Geometry: final body of the model. Coordinates: model frame, mm. Round coordinates to 2 decimals unless told otherwise and drop trailing zeros. Loops run counter-clockwise (first coordinate to the right, second up) from the corner with the lowest first, then second, coordinate; pieces in that order, holes last. Notation, with made-up numbers: M -33.75,-16 L 0.25,-16 A8 cw 0.25,-5 Z; hole C 38.5,-3.75 d6. An arc over 180 degrees is marked long. Answer as a JSON object with one key per item and string values.
```python
from build123d import *

# Parameters (mm, degrees)
SKETCH_W     = 20
SKETCH_H     = 30
PAD_DEPTH    = 2.5
SKETCH001_R  = 2.5
PAD001_DEPTH = 10
SKETCH002_R  = 3.75
PAD002_DEPTH = 3
FILLET_R     = 2
FILLET001_R  = 1.24


with BuildPart() as part:
    # Sketch → Pad (new body)
    with BuildSketch(Plane.XY):
        Rectangle(SKETCH_W, SKETCH_H)
    extrude(amount=PAD_DEPTH)

    # Sketch001 (on Face6 of Pad) → Pad001 (join)
    with BuildSketch(Plane.XY.offset(2.5)):
        Circle(SKETCH001_R)
    extrude(amount=PAD001_DEPTH)

    # Sketch002 (on Face8 of Pad001) → Pad002 (join)
    with BuildSketch(Plane.XY.offset(12.5)):
        Circle(SKETCH002_R)
    extrude(amount=PAD002_DEPTH)

    # Fillet
    fillet_edges = [part.edges().sort_by_distance(p)[0] for p in [
        (-10, 0, 2.5),
        (0, -15, 2.5),
        (10, 0, 2.5),
        (0, 15, 2.5),
        (-2.5, 0, 2.5),
    ]]
    fillet(fillet_edges, radius=FILLET_R)

    # Fillet001
    fillet001_edges = [part.edges().sort_by_distance(p)[0] for p in [
        (-3.75, 0, 12.5),
        (-3.75, 0, 15.5),
    ]]
    fillet(fillet001_edges, radius=FILLET001_R)


solid = part.part
```
1) Line query: probe 1 along Z at (x, y) = (7.5, 8.5); probe 2 along X at (y, z) = (0.5, 13.25); probe 3 along Z at (x, y) = (-8.5, 10.25). Output: solid intervals per line, ascending.
Geometry results:
{"probe 1": "0 to 2.5", "probe 2": "-3.61 to 3.61", "probe 3": "0 to 2.44"}
2) Pull-direction query (Z, two-part tool) for faces 1 (the face through (-9.4, 0.21, 1.93)), 2 (the face through (-0.54, -2.44, 8.44)), 3 (the face through (-3.746, 0.165, 13.996)), 4 (the face through (0, 0, 0)); classes: +Z half, -Z half, draft (parallel to the pull), parting line (faces both ways), or undercut.
Geometry results:
{"face 1": "+Z half", "face 2": "undercut", "face 3": "draft", "face 4": "-Z half"}
3) Cut plane C-C on z = 7.75. Return the cut outline in (x, y), and give its area (3 significant figures).
Geometry results:
{"outline": "C 0,0 d5", "area": "19.6 mm2"}
4) First-contact query: pin 1 (1 mm diameter, centred on x = -7.5, y = 11.5, fed in from -Z); pin 2 (4 mm diameter, centred on x = -1.5, z = 4, fed in from -Y). Flat tips, straight axial feed; report the tip coordinate or a pass-through.
Geometry results:
{"pin 1": "z = 0", "pin 2": "y = -14.32"}
5) Cut plane D-D on x = -5. Return the cut outline in (y, z).
Geometry results:
{"outline": "M -15,0 L 15,0 L 15,0.5 A2 ccw 13,2.5 L -13,2.5 A2 ccw -15,0.5 Z"}
